Input: dimensioned drawing with shaded views. Units: mm. Origin: part minimum x, y, z. A direction names the side the tool comes from. Round coordinates to 2 decimals unless told otherwise and drop trailing zeros. Write each loop counter-clockwise with the first axis right and the second up, starting at its lowest first coordinate (ties: lowest second). Pieces come first, ordered by that corner, then holes. Notation, with made-up numbers: (3.25, -20.75) -> (53.25, -20.75) arc R20 cw to (53.25, -2.75) -> close; hole circle Ø10 at (0.5, -39). An arc over 180 degrees is marked (long way). Use one line per item in the form item = value. Start each with the question number.
1. Cut plane A-A, the plane z = 4.5. Return the cut outline in (x, y).
2. Cut plane D-D, the plane z = 31. Return the cut outline in (x, y).
3. Cut plane B-B, the plane y = 62. Return the cut outline in (x, z), plus the area to 3 significant figures.
4. Pin query (flat end, axial travel): pin 1 Ø4 at (y, z) = (87.5, 38.5) entering from +X; pin 2 Ø17.5 at (y, z) = (54.5, 22.5) entering from +X; pin 3 Ø10 at (y, z) = (30, 13) entering from +X. Return the tip coordinate at first contact, or that it passes through.
5. Line query: L1, parallel to Y at x = 57, z = 4; L2, parallel to X at y = 36, z = 4.5; L3, parallel to Y at x = 61, z = 49. Output: solid intervals per line, ascending.
6. Reachability of the marked faces 1, 2 and 3 from +Z, -Z, +X, -X, +Y, -Y: full face, straight path, thin tool, end or side. Return the list, or none.
7. Cut plane C-C, the plane x = 25. Return the cut outline in (y, z), plus the area to 3 significant figures.
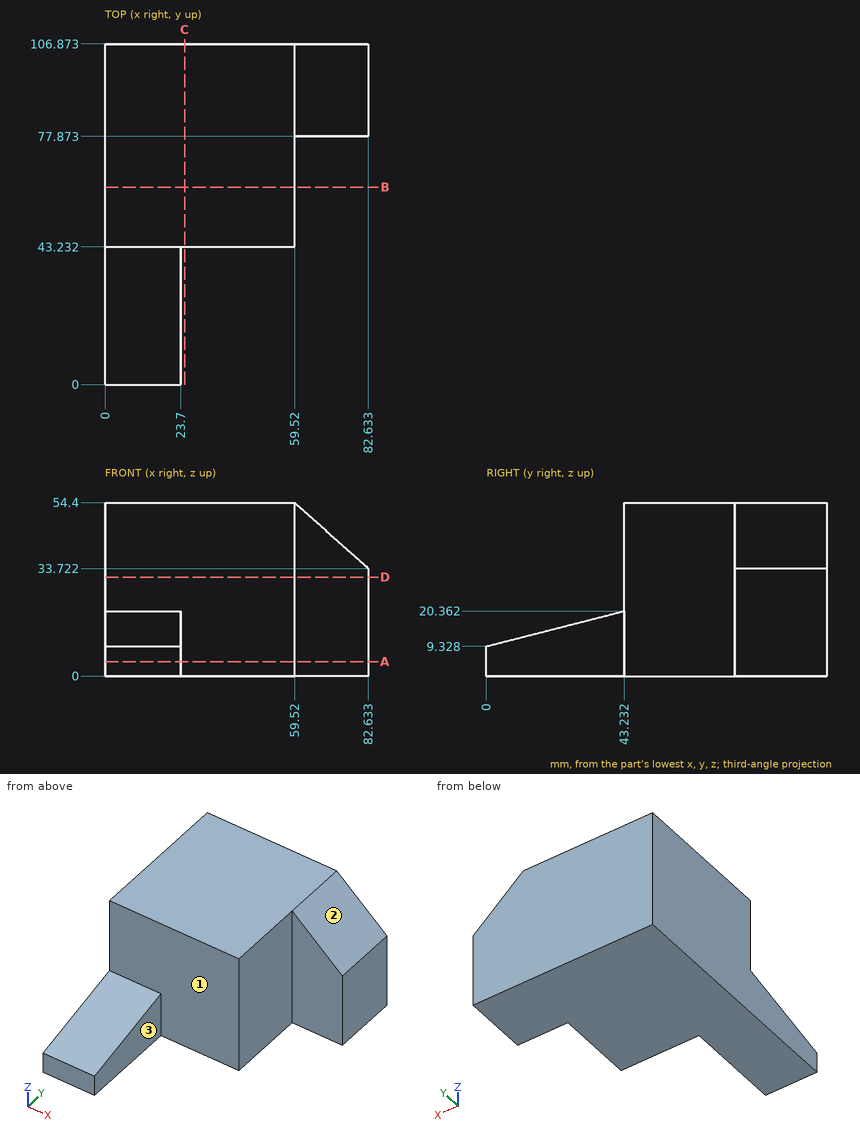
Outcome:
q1.outline = (0, 0) -> (23.7, 0) -> (23.7, 43.23) -> (59.52, 43.23) -> (59.52, 77.87) -> (82.63, 77.87) -> (82.63, 106.87) -> (0, 106.87) -> close
q2.outline = (0, 43.23) -> (59.52, 43.23) -> (59.52, 77.87) -> (82.63, 77.87) -> (82.63, 106.87) -> (0, 106.87) -> close
q3.outline = (0, 0) -> (59.52, 0) -> (59.52, 54.4) -> (0, 54.4) -> close
q3.area = 3,240 mm^2
q4.pin_1 = 79.53
q4.pin_2 = 59.52
q4.pin_3 = 23.7
q5.L1 = 43.23 to 106.87
q5.L2 = 0 to 23.7
q5.L3 = 77.87 to 106.87
q6.face_1 = +Z, +X, -Y
q6.face_2 = +Z, +X, +Y, -Y
q6.face_3 = +Z, -Z, +X, -Y
q7.outline = (43.23, 0) -> (106.87, 0) -> (106.87, 54.4) -> (43.23, 54.4) -> close
q7.area = 3,460 mm^2
